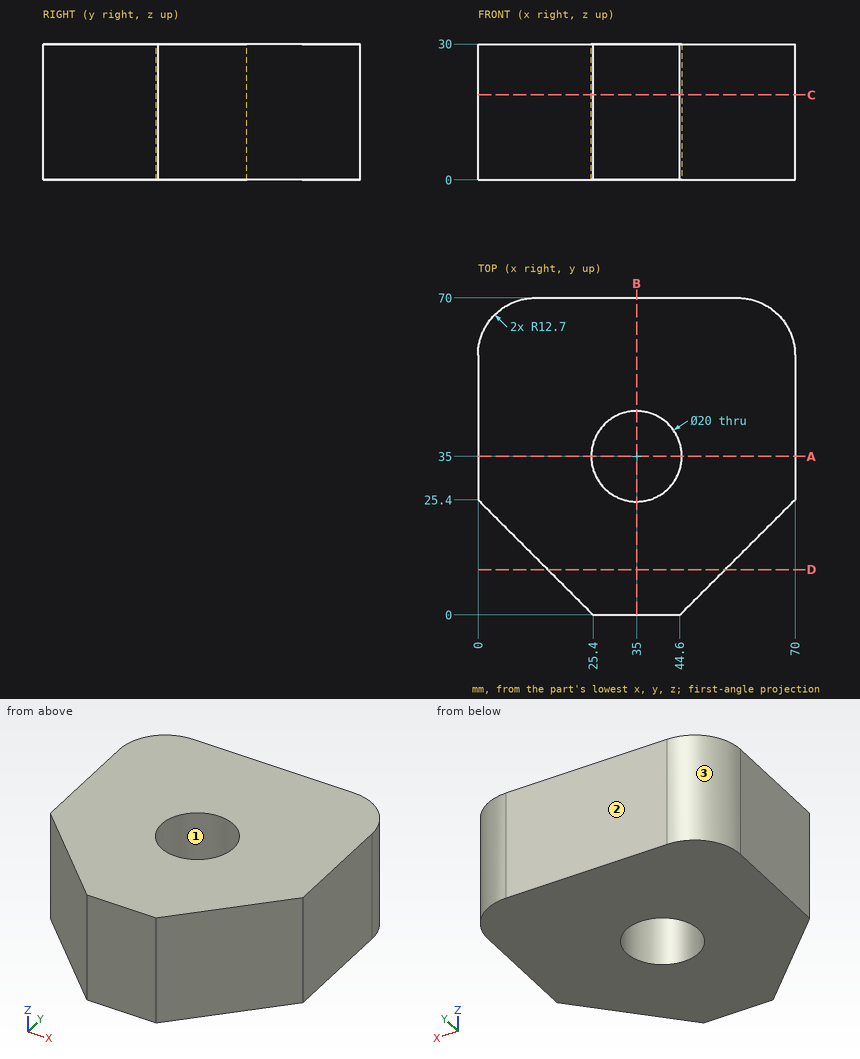
Answer from the drawing. Dimensions are ordinates in mm from the lowest x, y and z of the part. Coordinates: 2 decimals unless noted, no trailing zeros. Order: outer loops, then holes, each group sorted by start corner. A loop starts at its lowest first (then second) coordinate and runs counter-clockwise, first axis right, second up. Notation, with made-up numbers: M -21,8 L -3,8 A20 ccw -3,22 Z; hole C 6.25,88 d7. An arc over 180 degrees is marked long. Put each result on its own line as item: value. Start each with the question number.
Item 1: Section C-C, the plane z = 18.75 is taken. Determine the outline of the cut face in (x, y).
Item 2: The mould has two halves that part along X. Classify the marked faces 1, 2 and 3: +X half, -X half, draft (parallel to the pull), parting line (faces both ways), or undercut.
Item 3: Section D-D, the plane y = 10 is taken. Determine the outline of the cut face in (x, z), plus the area to 3 significant figures.
Item 4: Section A-A, the plane y = 35 is taken. Determine the outline of the cut face in (x, z).
Item 5: Given pin 1 Ø8 at (x, y) = (38.5, 25) entering from -Z; pin 2 Ø18 at (x, y) = (35, 35) entering from -Z; pin 3 Ø1.5 at (x, z) = (12.5, 20.5) entering from -Y; pin 4 Ø1 at (y, z) = (7, 9) entering from -X, each flat-ended and moving along its own axis, determine where each tip first touches the part or whether it passes through.
Item 6: Consider probe 1 along Y at (x, z) = (35, 19.25); probe 2 along Y at (x, z) = (31, 28.75); probe 3 along X at (y, z) = (37, 6). Determine where each line is inside the solid, lowest interval first. Write a range as [from, to].
Computed:
1. outline: M 0,25.4 L 25.4,0 L 44.6,0 L 70,25.4 L 70,57.3 A12.7 ccw 57.3,70 L 12.7,70 A12.7 ccw 0,57.3 Z; hole C 35,35 d20
2. face 1: undercut
2. face 2: draft
2. face 3: -X half
3. outline: M 15.4,0 L 54.6,0 L 54.6,30 L 15.4,30 Z
3. area: 1,180 mm2
4. outline: M 0,0 L 25,0 L 25,30 L 0,30 Z; M 45,0 L 70,0 L 70,30 L 45,30 Z
5. pin 1: stops at z = 0
5. pin 2: passes through
5. pin 3: stops at y = 12.15
5. pin 4: stops at x = 17.9
6. probe 1: y = [0, 25], [45, 70]
6. probe 2: y = [0, 25.83], [44.17, 70]
6. probe 3: x = [0, 25.2], [44.8, 70]
